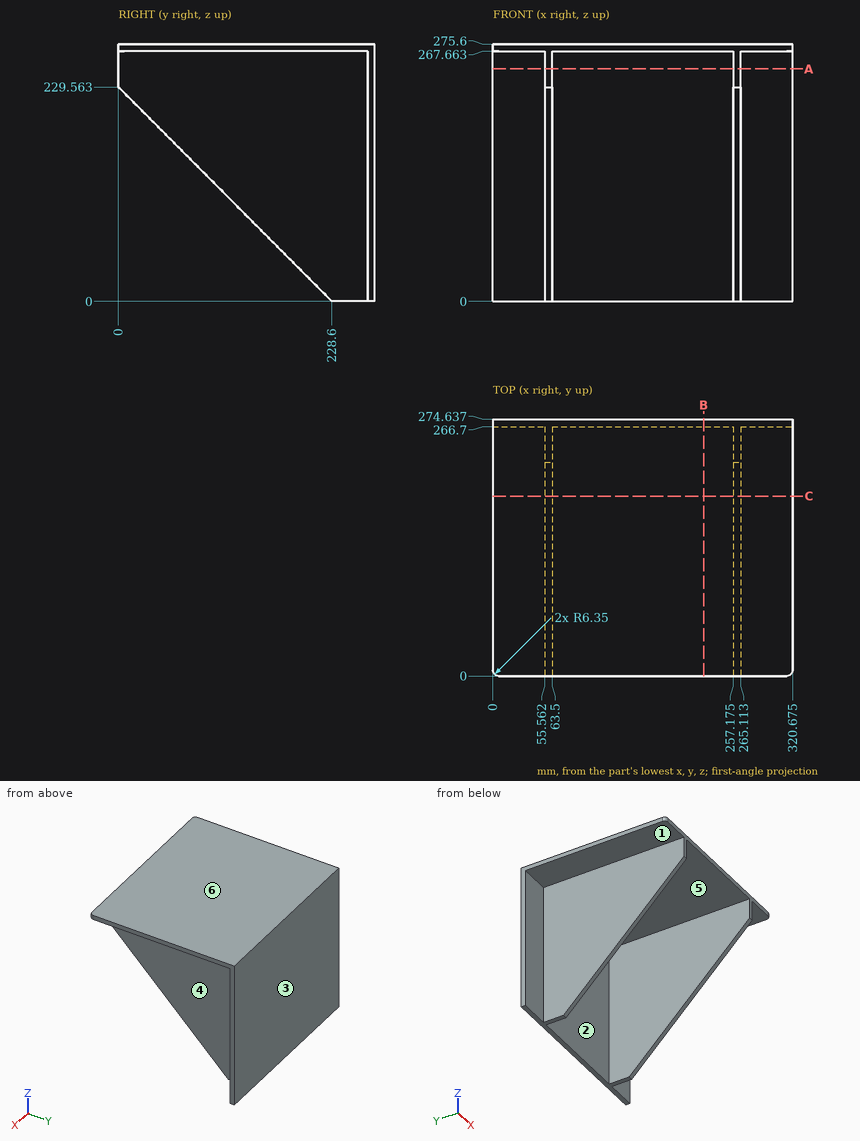
Here's the drawing with two shaded views (mm, measured from the low corner). I have some questions. A direction names the side the tool comes from. Round coordinates to 2 decimals unless told otherwise and drop trailing zeros. Loops run counter-clockwise (first coordinate to the right, second up) from the corner with the lowest first, then second, coordinate; pieces in that order, holes last.
Item 1: Please list where these lines run through material, in increasing order: L1, parallel to X at y = 239, z = 142 (1 decimal); L2, parallel to Z at x = 226.5, y = 23.5; L3, parallel to Y at x = 234.5, z = 166.5.
Item 2: Suppose I cut it at A-A, the plane z = 249. Write out the boundary of the cut face in (x, y) (1 decimal).
Item 3: Will these pins go through, and if not, where does the flat tip stop? pin 1 Ø3 at (y, z) = (224, 45) entering from -X; pin 2 Ø5 at (x, z) = (281, 68) entering from -Y.
Item 4: Suppose I cut it at B-B, the plane x = 225.5. Write out the boundary of the cut face in (y, z).
Item 5: If we mould it in two halves opening along X, with no side actions, what happens to the marked faces 4, 5 and 6? For each: +X half, -X half, draft (parallel to the pull), parting line (faces both ways), or undercut.
Item 6: Suppose I cut it at C-C, the plane y = 192.5. Write out the boundary of the cut face in (x, z) (1 decimal), then the cut area to 3 significant figures.
Item 7: Which directions (+Z, -Z, +X, -X, +Y, -Y) give clear straight access to the entire face, cutting with the end or side of a thin tool? Please do the marked faces 1, 2 and 3.
Reported:
1. L1: x = 55.6 to 63.5, 257.2 to 265.1
1. L2: z = 267.66 to 275.6
1. L3: y = 266.7 to 274.64
2. outline: (0, 266.7) - (55.6, 266.7) - (55.6, 0) - (63.5, 0) - (63.5, 266.7) - (257.2, 266.7) - (257.2, 0) - (265.1, 0) - (265.1, 266.7) - (320.7, 266.7) - (320.7, 274.6) - (0, 274.6) - close
3. pin 1: stops at x = 55.56
3. pin 2: stops at y = 266.7
4. outline: (0, 267.66) - (266.7, 267.66) - (266.7, 0) - (274.64, 0) - (274.64, 275.6) - (0, 275.6) - close
5. face 4: +X half
5. face 5: undercut
5. face 6: draft
6. outline: (0, 267.7) - (55.6, 267.7) - (55.6, 36.3) - (63.5, 36.3) - (63.5, 267.7) - (257.2, 267.7) - (257.2, 36.3) - (265.1, 36.3) - (265.1, 267.7) - (320.7, 267.7) - (320.7, 275.6) - (0, 275.6) - close
6. area: 6,220 mm2
7. face 1: -Z, -X, -Y
7. face 2: -Z, -Y
7. face 3: +Z, -Z, +X, -X, +Y
